Could you check a few things on this model? Use its own coordinates, in mm. Round coordinates to 2 decimals unless told otherwise and drop trailing zeros. Write each loop counter-clockwise with the first axis right and the second up, starting at its lowest first coordinate (ties: lowest second). Pieces come first, ordered by that corner, then holes. Notation, with made-up numbers: (-12.75, -19.75) -> (34.25, -19.75) arc R13 cw to (34.25, -8.75) -> close; hole circle Ø8 at (14, 77.25). An arc over 180 degrees is marked (long way). Return JSON: item names as keys, results as strings.
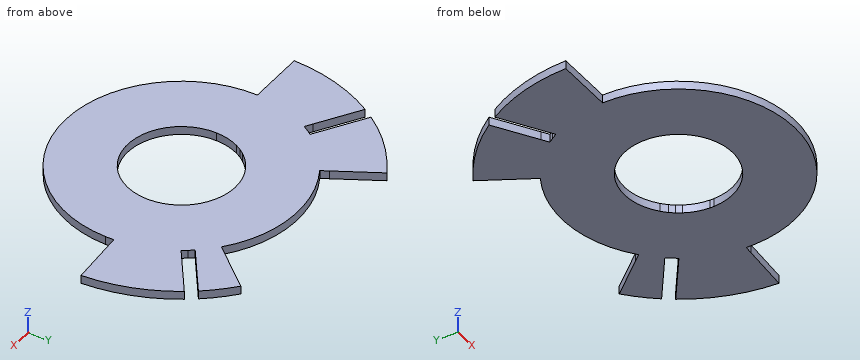
from build123d import *

# Parameters (mm, degrees)
F1_DEPTH = 1.4


# Not quite as in the source:
# - a feature names something its author has since deleted; it is built from what else it names


with BuildPart() as f1:
    # F0 (on Top) → F1 (new body)
    with BuildSketch(Plane.XY):
        with BuildLine():
            Line((9.1, 0), (19.6, 0))
            ThreePointArc((19.6, 0), (19.5880602096, 0.6840301354), (19.5522553851, 1.3672268854))
            Line((19.5522553851, 1.3672268854), (9.0778328574, 0.6347839111))
            ThreePointArc((9.0778328574, 0.6347839111), (9.0944565259, 0.31758542), (9.1, 0))
        make_face()
        with BuildLine():
            ThreePointArc((-19.6, 0), (0, -19.6), (19.6, 0))
            Line((19.6, 0), (9.1, 0))
            ThreePointArc((9.1, 0), (0, -9.1), (-9.1, 0))
            Line((-9.1, 0), (-19.6, 0))
        make_face()
        with BuildLine():
            Line((9.0778328574, 0.6347839111), (19.5522553851, 1.3672268854))
            ThreePointArc((19.5522553851, 1.3672268854), (18.5830433274, 6.2314124156), (16.4238667052, 10.6965696581))
            Line((16.4238667052, 10.6965696581), (7.9052534042, 4.5074348153))
            ThreePointArc((7.9052534042, 4.5074348153), (8.7095155433, 2.6371080753), (9.0778328574, 0.6347839111))
        make_face()
        with BuildLine():
            ThreePointArc((16.4238667052, 10.6965696581), (18.5830433274, 6.2314124156), (19.5522553851, 1.3672268854))
            Line((19.5522553851, 1.3672268854), (20.9488450555, 1.4648859486))
            ThreePointArc((20.9488450555, 1.4648859486), (19.8990062518, 6.7104061122), (17.5578688927, 11.5204704742))
            Line((17.5578688927, 11.5204704742), (16.4238667052, 10.6965696581))
        make_face()
        with BuildLine():
            Line((-21, 0), (-19.6, 0))
            ThreePointArc((-19.6, 0), (-18.9724573243, 4.9199454342), (-17.1300139719, 9.5248423254))
            Line((-17.1300139719, 9.5248423254), (-18.3187262027, 10.2676321667))
            ThreePointArc((-18.3187262027, 10.2676321667), (-20.3186275405, 5.3059753931), (-21, 0))
        make_face()
        with BuildLine():
            ThreePointArc((-17.1300139719, 9.5248423254), (-18.9724573243, 4.9199454342), (-19.6, 0))
            Line((-19.6, 0), (-9.1, 0))
            ThreePointArc((-9.1, 0), (-8.8722549614, 2.0231391203), (-8.2004193626, 3.9450123291))
            Line((-8.2004193626, 3.9450123291), (-17.1300139719, 9.5248423254))
        make_face()
        with BuildLine():
            Line((7.9052534042, 4.5074348153), (16.4238667052, 10.6965696581))
            ThreePointArc((16.4238667052, 10.6965696581), (16.1455577033, 11.1121989925), (15.8567330897, 11.5205909449))
            Line((15.8567330897, 11.5205909449), (7.3620546488, 5.3488457959))
            ThreePointArc((7.3620546488, 5.3488457959), (7.6452381851, 4.9356188157), (7.9052534042, 4.5074348153))
        make_face()
        with BuildLine():
            ThreePointArc((17.5578688927, 11.5204704742), (19.8990062518, 6.7104061122), (20.9488450555, 1.4648859486))
            Line((20.9488450555, 1.4648859486), (29.0291138626, 2.029913386))
            ThreePointArc((29.0291138626, 2.029913386), (27.512052622, 9.481400768), (24.1162750467, 16.285431461))
            Line((24.1162750467, 16.285431461), (17.5578688927, 11.5204704742))
        make_face()
        with BuildLine():
            ThreePointArc((-16.6217426847, 10.386417579), (-16.8813757535, 9.9588730623), (-17.1300139719, 9.5248423254))
            Line((-17.1300139719, 9.5248423254), (-8.2004193626, 3.9450123291))
            ThreePointArc((-8.2004193626, 3.9450123291), (-7.9709061334, 4.3902910396), (-7.717237675, 4.8222653045))
            Line((-7.717237675, 4.8222653045), (-16.6217426847, 10.386417579))
        make_face()
        with BuildLine():
            Line((-29.1, 0), (-21, 0))
            ThreePointArc((-21, 0), (-20.3186275405, 5.3059753931), (-18.3187262027, 10.2676321667))
            Line((-18.3187262027, 10.2676321667), (-25.1935432849, 14.5634946614))
            ThreePointArc((-25.1935432849, 14.5634946614), (-28.1064237283, 7.5391607759), (-29.1, 0))
        make_face()
        with BuildLine():
            Line((7.3620546488, 5.3488457959), (15.8567330897, 11.5205909449))
            ThreePointArc((15.8567330897, 11.5205909449), (15.5575809762, 11.9214795294), (15.2482962006, 12.3146036469))
            Line((15.2482962006, 12.3146036469), (6.7296828997, 6.1254688041))
            ThreePointArc((6.7296828997, 6.1254688041), (7.0565609618, 5.7458635027), (7.3620546488, 5.3488457959))
        make_face()
        with BuildLine():
            ThreePointArc((-16.0701754434, 11.2209385177), (-16.3512838646, 10.8071974155), (-16.6217426847, 10.386417579))
            Line((-16.6217426847, 10.386417579), (-7.717237675, 4.8222653045))
            ThreePointArc((-7.717237675, 4.8222653045), (-7.4401827106, 5.2396260586), (-7.1405808342, 5.6411085215))
            Line((-7.1405808342, 5.6411085215), (-16.0701754434, 11.2209385177))
        make_face()
        with BuildLine():
            Line((6.7296828997, 6.1254688041), (15.2482962006, 12.3146036469))
            ThreePointArc((15.2482962006, 12.3146036469), (13.9887542441, 13.7286108073), (12.5986371499, 15.0144710851))
            Line((12.5986371499, 15.0144710851), (5.8493672481, 6.9710044324))
            ThreePointArc((5.8493672481, 6.9710044324), (6.3037178141, 6.5630131586), (6.7296828997, 6.1254688041))
        make_face()
        with BuildLine():
            ThreePointArc((12.5986371499, 15.0144710851), (13.9887542441, 13.7286108073), (15.2482962006, 12.3146036469))
            Line((15.2482962006, 12.3146036469), (16.3822983881, 13.1385044629))
            ThreePointArc((16.3822983881, 13.1385044629), (15.0129754185, 14.6836837709), (13.4985398034, 16.0869333055))
            Line((13.4985398034, 16.0869333055), (12.5986371499, 15.0144710851))
        make_face()
        with BuildLine():
            Line((-17.2588876742, 11.963728359), (-16.0701754434, 11.2209385177))
            ThreePointArc((-16.0701754434, 11.2209385177), (-13.2510831681, 14.4419110533), (-9.8, 16.9740979142))
            Line((-9.8, 16.9740979142), (-10.5, 18.1865334795))
            ThreePointArc((-10.5, 18.1865334795), (-14.2239160262, 15.4492787172), (-17.2588876742, 11.963728359))
        make_face()
        with BuildLine():
            ThreePointArc((-9.8, 16.9740979142), (-13.2510831681, 14.4419110533), (-16.0701754434, 11.2209385177))
            Line((-16.0701754434, 11.2209385177), (-7.1405808342, 5.6411085215))
            ThreePointArc((-7.1405808342, 5.6411085215), (-5.9515972184, 6.8839298769), (-4.55, 7.8808311744))
            Line((-4.55, 7.8808311744), (-9.8, 16.9740979142))
        make_face()
        with BuildLine():
            Line((5.8493672481, 6.9710044324), (12.5986371499, 15.0144710851))
            ThreePointArc((12.5986371499, 15.0144710851), (1.7082525579, 19.5254160826), (-9.8, 16.9740979142))
            Line((-9.8, 16.9740979142), (-4.55, 7.8808311744))
            ThreePointArc((-4.55, 7.8808311744), (0.793117259, 9.0653717526), (5.8493672481, 6.9710044324))
        make_face()
        with BuildLine():
            ThreePointArc((13.4985398034, 16.0869333055), (15.0129754185, 14.6836837709), (16.3822983881, 13.1385044629))
            Line((16.3822983881, 13.1385044629), (22.9407045421, 17.9034654498))
            ThreePointArc((22.9407045421, 17.9034654498), (20.9382004615, 20.2089525071), (18.7051194419, 22.2918932948))
            Line((18.7051194419, 22.2918932948), (13.4985398034, 16.0869333055))
        make_face()
        with BuildLine():
            Line((-24.1337047564, 16.2595908537), (-17.2588876742, 11.963728359))
            ThreePointArc((-17.2588876742, 11.963728359), (-14.2239160262, 15.4492787172), (-10.5, 18.1865334795))
            Line((-10.5, 18.1865334795), (-14.55, 25.2013392501))
            ThreePointArc((-14.55, 25.2013392501), (-19.8518505313, 21.2770775832), (-24.1337047564, 16.2595908537))
        make_face()
    extrude(amount=F1_DEPTH)


solid = f1.part
1) I want a section at B-B, the plane y = 21. Please give me the cut outline in (x, z), and give its area (3 significant figures).
Return value:
{"outline": "(-20.14, 0) -> (-12.12, 0) -> (-12.12, 1.4) -> (-20.14, 1.4) -> close; (17.62, 0) -> (20.14, 0) -> (20.14, 1.4) -> (17.62, 1.4) -> close", "area": "14.8 mm²"}
2) I want a section at D-D, the plane y = -11. Please give me the cut outline in (x, z), and give its area (3 significant figures).
Return value:
{"outline": "(-16.22, 0) -> (16.22, 0) -> (16.22, 1.4) -> (-16.22, 1.4) -> close", "area": "45.4 mm²"}
3) I want a section at C-C, the plane x = 12. Please give me the cut outline in (y, z).
Return value:
{"outline": "(-15.5, 0) -> (15.5, 0) -> (15.5, 1.4) -> (-15.5, 1.4) -> close"}
4) Will this pin go through, and if not, where does the flat tip stop? pin 1 Ø0.7 at (x, z) = (-23.5, 1) entering from -Y.
Return value:
{"pin 1": "y = 0"}
5) If I drill on probe 1 along X at (y, z) = (18, 0.9); probe 2 along X at (y, z) = (15.5, 1.3); probe 3 along X at (y, z) = (-3, 0.25), over which ranges is the centre line in solid material (lowest first)? Write a range as [from, to].
Return value:
{"probe 1": "[-22.87, -10.39], [-7.76, 7.76], [15.1, 22.87]", "probe 2": "[-22.92, 12], [13.01, 19.63], [23.04, 24.63]", "probe 3": "[-19.37, -8.59], [8.59, 19.37]"}
6) I want a section at A-A, the plane x = 0. Please give me the cut outline in (y, z).
Return value:
{"outline": "(-19.6, 0) -> (-9.1, 0) -> (-9.1, 1.4) -> (-19.6, 1.4) -> close; (9.1, 0) -> (19.6, 0) -> (19.6, 1.4) -> (9.1, 1.4) -> close"}
